Geometry: final body of the model. Coordinates: model frame, mm. Face numbers are marked on the shaded views. Coordinates: 2 decimals unless noted, no trailing zeros. Order: outer loops, then holes, each group sorted by start corner. A loop starts at its lowest first (then second) coordinate and runs counter-clockwise, first axis right, second up. Notation, with made-up numbers: M 66.25,10.5 L 71.25,10.5 A19 ccw 71.25,27.5 Z; hole C 61,84 d8. An arc over 180 degrees is marked long. Use CSV: the item, a comma, the result in double quotes. Start each with the question number.
1. Section query D-D on z = 8. Return the cut outline in (x, y), and give its area (3 significant figures).
2. Material intervals for line 1 (Y direction, x = 4, z = 0); line 2 (X direction, y = -4.75, z = 11.25); line 3 (Z direction, x = 3, y = -2.5), sorted ascending.
3. Pull-direction query (Z, two-part tool) for the marked faces 1, 2 and 3; classes: pulls with the +Z half, pulls with the -Z half, needs draft (parallel to the pull), parting line crosses it, or undercut.
4. Section query B-B on y = -12. Return the cut outline in (x, z).
5. Section query A-A on z = -2.5. Return the cut outline in (x, y).
6. Section query C-C on x = 8.5. Return the cut outline in (y, z), and give its area (3 significant figures).
7. First-contact query: P1, Ø5, axis at y = 8.85, z = -7.42, coming from the +X side; P2, Ø2.5, axis at y = -5.78, z = 10, coming from the +X side; P3, Ø5, axis at x = 10.5, z = 5, coming from the -Y side; P4, Ø3, axis at x = 8.5, y = 0, coming from the +Z side. Flat tips, straight axial feed; report the tip coordinate or a pass-through.
from build123d import *

# Parameters (mm, degrees)
SKETCH1_W                      = 1.4
SKETCH1_H                      = 15
SKETCH2_R                      = 6.95
BOSS_EXTRUDE1_DEPTH            = 11.1
F_4_0_4_DIAMETER_HOLE1_D       = 4
F_4_0_4_DIAMETER_HOLE1_DEPTH   = 1.4
F_2_9_2_9_DIAMETER_HOLE1_D     = 2.9
F_2_9_2_9_DIAMETER_HOLE1_DEPTH = 1.4
F_9_0_9_DIAMETER_HOLE1_D       = 9
F_9_0_9_DIAMETER_HOLE1_DEPTH   = 12.5
SKETCH9_W                      = 1.25
SKETCH9_H                      = 10.677095884
F_2_5_2_5_DIAMETER_HOLE2_D     = 2.5
F_2_5_2_5_DIAMETER_HOLE2_DEPTH = 10.677095884


with BuildPart() as part:
    # Sketch1 → Revolve1 (revolve)
    with BuildSketch(Plane.XY):
        with Locations((0.7, 7.5)):
            Rectangle(SKETCH1_W, SKETCH1_H)
    revolve(axis=Axis((0, 0, 0), (1, 0, 0)))

    # Sketch2 → Boss-Extrude1 (add)
    with BuildSketch(Plane(origin=(1.4, 0, 0), x_dir=(0, 0, -1), z_dir=(1, 0, 0))):
        Circle(SKETCH2_R)
    extrude(amount=BOSS_EXTRUDE1_DEPTH)

    # Ø4.0 (4) Diameter Hole1
    with Locations(Plane(origin=(1.4, 0, 0), x_dir=(0, 0, -1), z_dir=(1, 0, 0))):
        with Locations((-7.424196892, 8.847813318), (-11.374529547, 2.005636452), (-3.950332655, -10.85344977), (3.950332655, -10.85344977), (11.374529547, 2.005636452), (7.424196892, 8.847813318)):
            Hole(F_4_0_4_DIAMETER_HOLE1_D / 2, depth=F_4_0_4_DIAMETER_HOLE1_DEPTH)

    # Ø2.9 (2.9) Diameter Hole1
    with Locations(Plane(origin=(1.4, 0, 0), x_dir=(0, 0, -1), z_dir=(1, 0, 0))):
        with Locations((0, 11.55), (-10.002593414, -5.775), (10.002593414, -5.775)):
            Hole(F_2_9_2_9_DIAMETER_HOLE1_D / 2, depth=F_2_9_2_9_DIAMETER_HOLE1_DEPTH)

    # Ø9.0 (9) Diameter Hole1
    with Locations(Plane.ZY):
        with Locations((0, 0)):
            Hole(F_9_0_9_DIAMETER_HOLE1_D / 2, depth=F_9_0_9_DIAMETER_HOLE1_DEPTH)

    # Sketch9 → Ø2.5 (2.5) Diameter Hole1 (revolve, cut)
    with BuildSketch(Plane(origin=(8.5, 0, -4.322904116), x_dir=(0, -1, 0), z_dir=(1, 0, 0))):
        with Locations((0.625, 5.338547942)):
            Rectangle(SKETCH9_W, SKETCH9_H)
    revolve(axis=Axis((8.5, 0, 2.027095884), (0, 0, -1)), mode=Mode.SUBTRACT)

    # Ø2.5 (2.5) Diameter Hole2
    with Locations(Plane(origin=(0, 0, 4.322904116), x_dir=(-1, 0, 0), z_dir=(0, 0, -1))):
        with Locations((-8.5, 0)):
            Hole(F_2_5_2_5_DIAMETER_HOLE2_D / 2, depth=F_2_5_2_5_DIAMETER_HOLE2_DEPTH)


solid = part.part
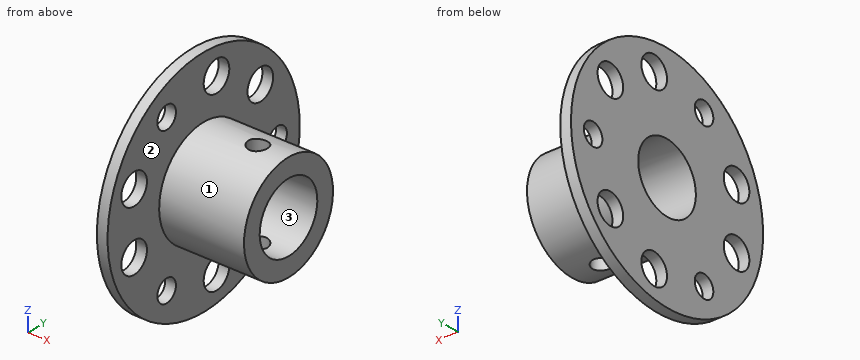
Results list:
1,outline,"M 0,-12.69 L 1.4,-12.69 L 1.4,6.93 L 0,6.93 Z; M 0,10.76 L 1.4,10.76 L 1.4,12.69 L 0,12.69 Z"
1,area,"30.2 mm²"
2,line 1,"y = -6.95 to -4.5, 4.5 to 6.95"
2,line 2,"x = 0 to 1.4"
2,line 3,"z = -6.48 to -3.74, 3.74 to 6.48"
3,face 1,"parting line crosses it"
3,face 2,"needs draft"
3,face 3,"undercut"
4,outline,"M 0,-9 L 1.4,-9 L 1.4,-5.59 L 0,-5.59 Z; M 0,-2.31 L 1.4,-2.31 L 1.4,2.31 L 0,2.31 Z; M 0,5.59 L 1.4,5.59 L 1.4,9 L 0,9 Z"
5,outline,"M 0,-14.79 L 1.4,-14.79 L 1.4,-12.23 L 0,-12.23 Z; M 0,-9.48 L 1.4,-9.48 L 1.4,-6.48 L 12.5,-6.48 L 12.5,-3.74 L 0,-3.74 Z; M 0,3.74 L 12.5,3.74 L 12.5,6.48 L 1.4,6.48 L 1.4,14.79 L 0,14.79 Z"
6,outline,"M -1.25,-6.84 L -1.25,-4.32 A4.5 cw -1.25,4.32 L -1.25,6.84 A6.95 ccw Z; M 1.25,-6.84 A6.95 ccw 1.25,6.84 L 1.25,4.32 A4.5 cw 1.25,-4.32 Z"
6,area,"75.8 mm²"
7,P1,"stops at x = 1.4"
7,P2,"passes through"
7,P3,"stops at y = -6.48"
7,P4,"stops at z = 6.95"
